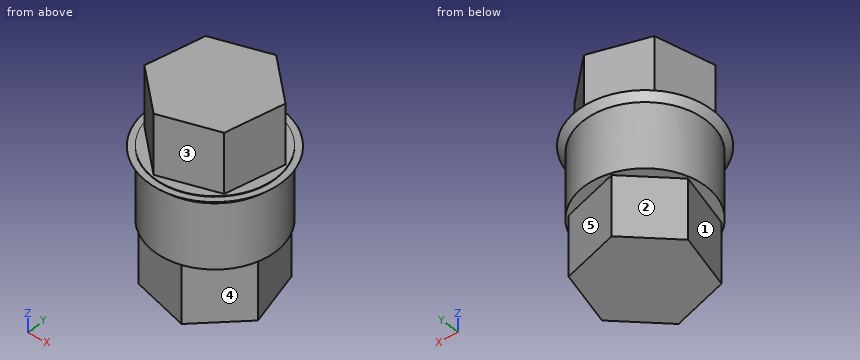
```python
from build123d import *

# Parameters (mm, degrees)
SKETCH_R     = 5.03
PAD_DEPTH    = 6
PAD001_DEPTH = 5
PAD002_DEPTH = 5


with BuildPart() as part:
    # Sketch → Pad (new body)
    with BuildSketch(Plane.XY):
        Circle(SKETCH_R)
    extrude(amount=PAD_DEPTH)

    # Sketch001 → Revolution (revolve)
    with BuildSketch(Plane.XZ):
        Polygon((4.824, 5.954), (5.562116, 5.954), (4.824, 5.204), align=None)
    revolve(axis=Axis((0, 0, 0), (0, 0, 1)))

    # Sketch002 (on Face6 of Revolution) → Pad001 (join)
    with BuildSketch(Plane.XY.offset(6)):
        Polygon((3.583031, -3.253843), (4.609426, 1.476074), (1.026395, 4.729917), (-3.583031, 3.253843), (-4.609426, -1.476074), (-1.026395, -4.729917), align=None)
    extrude(amount=PAD001_DEPTH)

    # Sketch003 (on Face2 of Pad001) → Pad002 (join)
    with BuildSketch(Plane(origin=(0, 0, 0), x_dir=(1, 0, 0), z_dir=(0, 0, -1))):
        Polygon((3.424679, -3.420114), (4.674245, 1.255802), (1.249566, 4.675915), (-3.424679, 3.420114), (-4.674245, -1.255802), (-1.249566, -4.675915), align=None)
    extrude(amount=PAD002_DEPTH)


solid = part.part
```
CAD build for the part. Positions are in the model's coordinates, mm. Face numbers are marked on the shaded views. A direction names the side the tool comes from. Give positions to 0.01 mm unless a question says otherwise; leave off trailing zeros. Loops run counter-clockwise (first coordinate to the right, second up) from the corner with the lowest first, then second, coordinate; pieces in that order, holes last. Notation, with made-up numbers: M 74.25,-18.5 L 122.25,-18.5 A35 cw 122.25,15.5 Z; hole C 28,64.25 d6. An arc over 180 degrees is marked long. Use one line per item in the form item = value.
Item 1: Flat gauge pins, fed straight in: pin 1 (5 mm diameter, centred on y = 3.5, z = -2.5, fed in from +X); pin 2 (4 mm diameter, centred on x = -2.5, z = 2, fed in from -Y). Where does each tip first touch, or does it go through?
Determined:
pin_1 = 4.07
pin_2 = -5.01
Item 2: Which spindle directions (+Z, -Z, +X, -X, +Y, -Y) get a long thin tool onto all of the face, cutting with end or side? Do the marked faces 1, 2, 3, 4 and 5. Say none if no direction does.
Determined:
face_1 = -Z, -X, -Y
face_2 = -Z, -X, +Y
face_3 = +Z, +X, -Y
face_4 = -Z, +X, -Y
face_5 = -Z, +X, +Y
Item 3: Drill centre lines: probe 1 along Z at (x, y) = (-3, -3); probe 2 along Z at (x, y) = (0.5, -4.75); probe 3 along X at (y, z) = (0.75, 0.75). Where is each one in solid material? Low to high. Write a range as from..to.
Determined:
probe_1 = -5..6
probe_2 = 0..6
probe_3 = -4.97..4.97
Item 4: Slice it at C-C (y = 0). List the corners of the cut face in (x, z).
Determined:
outline = M -5.56,5.95 L -5.03,5.41 L -5.03,0 L -4.34,0 L -4.34,-5 L 4.34,-5 L 4.34,0 L 5.03,0 L 5.03,5.41 L 5.56,5.95 L 5.03,5.95 L 5.03,6 L 4.29,6 L 4.29,11 L -4.29,11 L -4.29,6 L -5.03,6 L -5.03,5.95 Z
Item 5: Slice it at A-A (z = 10.25). List the corners of the cut face in (x, y), plus the area to 3 significant figures.
Determined:
outline = M -4.61,-1.48 L -1.03,-4.73 L 3.58,-3.25 L 4.61,1.48 L 1.03,4.73 L -3.58,3.25 Z
area = 60.9 mm2
Item 6: Slice it at D-D (z = 5). List the corners of the cut face in (x, y), plus the area to 3 significant figures.
Determined:
outline = C 0,0 d10.06
area = 79.5 mm2
Item 7: Slice it at B-B (x = 0). List the corners of the cut face in (y, z).
Determined:
outline = M -5.56,5.95 L -5.03,5.41 L -5.03,0 L -4.34,0 L -4.34,-5 L 4.34,-5 L 4.34,0 L 5.03,0 L 5.03,5.41 L 5.56,5.95 L 5.03,5.95 L 5.03,6 L 4.4,6 L 4.4,11 L -4.4,11 L -4.4,6 L -5.03,6 L -5.03,5.95 Z
